```python
from build123d import *

# Parameters (mm, degrees)
F0_R     = 12.5
F1_DEPTH = 25
F3_DEPTH = 25
F4_R     = 5


with BuildPart() as f1:
    # F0 (on Front) → F1 (new body)
    with BuildSketch(Plane.XZ):
        with BuildLine():
            ThreePointArc((24.534938, -13.386702), (27.082309, -6.907643), (27.949365, 0))
            ThreePointArc((27.949365, 0), (12.18024, 25.15569), (-17.333149, 21.925531))
            ThreePointArc((-17.333149, 21.925531), (-18.01957, -21.364973), (24.534938, -13.386702))
        make_face()
        Circle(F0_R, mode=Mode.SUBTRACT)
        with BuildLine():
            ThreePointArc((-17.333149, 21.925531), (12.18024, 25.15569), (27.949365, 0))
            ThreePointArc((27.949365, 0), (27.082309, -6.907643), (24.534938, -13.386702))
            Line((24.534938, -13.386702), (54.946235, 42.350645))
            ThreePointArc((54.946235, 42.350645), (32.107876, 38.068828), (32.476267, 61.302185))
            Line((32.476267, 61.302185), (-17.333149, 21.925531))
        make_face()
        with BuildLine():
            ThreePointArc((56.778706, 49.535085), (48.315655, 63.035762), (32.476267, 61.302185))
            ThreePointArc((32.476267, 61.302185), (32.107876, 38.068828), (54.946235, 42.350645))
            ThreePointArc((54.946235, 42.350645), (56.31337, 45.827858), (56.778706, 49.535085))
        make_face()
    extrude(amount=F1_DEPTH)

    # F2 (on face) → F3 (cut)
    with BuildSketch(Plane(origin=(24.534938, 0, -13.386702), x_dir=(0, 1, 0), z_dir=(0.877835, 0, -0.478963))):
        Polygon((-19.126982, 31.178041), (-10.197443, 46.199725), (-21.724535, 59.334177), (-25, 57.925509), (-25, 32.504715), align=None)
    extrude(amount=-F3_DEPTH, mode=Mode.SUBTRACT)

    # F4
    f4_edges = [f1.edges().sort_by_distance(p)[0] for p in [
        (7.571559, -25, 41.613858),
    ]]
    fillet(f4_edges, radius=F4_R)


solid = f1.part
```
Verification items for the finished model (mm, model axes). A direction names the side the tool comes from. Round coordinates to 2 decimals unless told otherwise and drop trailing zeros. Order: outer loops, then holes, each group sorted by start corner. A loop starts at its lowest first (then second) coordinate and runs counter-clockwise, first axis right, second up. Notation, with made-up numbers: (62.5, -35.75) -> (108.5, -35.75) arc R14 cw to (108.5, -17.75) -> close; hole circle Ø3 at (48, 53.5). An arc over 180 degrees is marked (long way). Put each result on its own line as item: value. Start each with the question number.
(1) Section check C-C (y = -17.5). Enter the section's corners in (x, z), then the cut area to 3 significant figures.
(2) Section check A-A (y = -5.5). Enter the section's corners in (x, z), then the cut area to 3 significant figures.
(3) Material ranges on line 1 along Z through (x, y) = (2.5, -9.5); line 2 along Z through (x, y) = (0, -11.5); line 3 along X through (y, z) = (-22.75, -11), recorded low to high.
(4) Depth check by flat-ended pin: pin 1 Ø5 at (x, y) = (-9, -6) entering from +Z; pin 2 Ø12 at (x, y) = (-15, -7) entering from +Z; pin 3 Ø5 at (x, y) = (35, -13.5) entering from +Z. Enter the tip coordinate at first touch or a pass-through.
(5) Section check B-B (y = -12). Enter the section's corners in (x, z).
(6) Draft check along X on faces 1 (the face through (-18.544, -9.86, -20.911)), 2 (the face through (32.2, -14.72, 26.39)), 3 (the face through (31.177, -23.496, 1.763)). Enter one of: +X half, -X half, draft (parallel to the pull), parting line (faces both ways), or undercut.
(7) Tool access check on faces 4 (the face through (41.665, -23.339, 44.067)), 5 (the face through (8.11, -23.5, 40.22)), 6 (the face through (28.971, -22.105, 20.476)). Record the directions out of +Z, -Z, +X, -X, +Y, -Y that give a thin tool (end or side, any length) a straight path to the whole face; none if there is none.
Completed:
1. outline: (-17.33, 21.93) arc R27.95 ccw (long way) to (24.53, -13.39) -> (40.78, 16.39) -> (18.83, 28.36) -> (28.7, 46.45) -> (50.65, 34.47) -> (54.95, 42.35) arc R15 ccw to (56.78, 49.54) arc R15 ccw to (32.48, 61.3) -> close; hole circle Ø25 at (0, 0)
1. area: 3,410 mm2
2. outline: (-17.33, 21.93) arc R27.95 ccw (long way) to (24.53, -13.39) -> (54.95, 42.35) arc R15 ccw to (56.78, 49.54) arc R15 ccw to (32.48, 61.3) -> close; hole circle Ø25 at (0, 0)
2. area: 3,930 mm2
3. line 1: z = -27.84 to -12.25, 12.25 to 37.6
3. line 2: z = -27.95 to -12.5, 12.5 to 35.63
3. line 3: x = -24.79 to -5.94, 5.94 to 24.9
4. pin 1: stops at z = 30.49
4. pin 2: stops at z = 28.51
4. pin 3: stops at z = 63.91
5. outline: (-17.33, 21.93) arc R27.95 ccw (long way) to (24.53, -13.39) -> (45.21, 24.51) -> (23.26, 36.48) -> (25.7, 40.95) -> (47.65, 28.97) -> (54.95, 42.35) arc R15 ccw to (56.78, 49.54) arc R15 ccw to (32.48, 61.3) -> close; hole circle Ø25 at (0, 0)
6. face 1: parting line
6. face 2: undercut
6. face 3: +X half
7. face 4: none
7. face 5: +Z, -X, -Y
7. face 6: +X
